from build123d import *

# Parameters (mm, degrees)
BOSS_EXTRUDE1_DEPTH = 20
MOVE_FACE1_BY       = 10
MOVE_FACE2_BY       = 10
SKETCH2_R           = 0.75
CUT_EXTRUDE1_DEPTH  = 88.464278423
SKETCH3_R           = 0.75
CUT_EXTRUDE2_DEPTH  = 108.819293264
SKETCH5_R           = 3.175
CUT_EXTRUDE3_DEPTH  = 88.464278423


with BuildPart() as part:
    # Sketch1 → Boss-Extrude1 (new, symmetric)
    with BuildSketch(Plane.XY):
        Polygon((0, 0), (-40, 0), (-40, 4), (-5, 4), (-5, 55), (50, 55), (50, 50), (0, 50), align=None)
    extrude(amount=BOSS_EXTRUDE1_DEPTH, both=True)

    # Move Face1: a face moved outward by 10.0
    extrude(part.faces().sort_by_distance((22.5, 55, 0))[0], amount=MOVE_FACE1_BY, dir=(0, 1, 0))

    # Move Face2: a face moved inward by 10.0
    extrude(part.faces().sort_by_distance((25, 50, 0))[0], amount=MOVE_FACE2_BY, dir=(0, 1, 0), mode=Mode.SUBTRACT)

    # Sketch2 → Cut-Extrude1 (cut, through all)
    with BuildSketch(Plane.ZY.offset(5)):
        with Locations((-10, 22)):
            Circle(SKETCH2_R)
        with Locations((10, 22)):
            Circle(SKETCH2_R)
        with Locations((10, 47)):
            Circle(SKETCH2_R)
        with Locations((-10, 47)):
            Circle(SKETCH2_R)
    extrude(amount=-CUT_EXTRUDE1_DEPTH, mode=Mode.SUBTRACT)

    # Sketch3 → Cut-Extrude2 (cut, through all)
    with BuildSketch(Plane(origin=(0, 65, -50), x_dir=(1, 0, 0), z_dir=(0, -1, 0))):
        with Locations(Location((10, 39.375, 0), (0, 0, 180))):
            Circle(SKETCH3_R)
        with Locations(Location((35, 39.375, 0), (0, 0, 90))):
            Circle(SKETCH3_R)
        with Locations(Location((35, 60.625, 0), (0, 0, 180))):
            Circle(SKETCH3_R)
        with Locations(Location((10, 60.625, 0), (0, 0, 90))):
            Circle(SKETCH3_R)
    extrude(amount=CUT_EXTRUDE2_DEPTH, mode=Mode.SUBTRACT)

    # Sketch5 → Cut-Extrude3 (cut, through all)
    with BuildSketch(Plane.ZY.offset(5)):
        with Locations(Location((0, 35, 0), (0, 0, 270))):
            Circle(SKETCH5_R)
    extrude(amount=-CUT_EXTRUDE3_DEPTH, mode=Mode.SUBTRACT)


solid = part.part
Could you check a few things on this model? Use its own coordinates, in mm. A direction names the side the tool comes from. Round coordinates to 2 decimals unless told otherwise and drop trailing zeros. Order: outer loops, then holes, each group sorted by start corner. A loop starts at its lowest first (then second) coordinate and runs counter-clockwise, first axis right, second up.
(1) Imagine slicing it at C-C (x = 2). Write out the boundary of the cut face in (y, z), plus the area to 3 significant figures.
Response values:
outline: (60, -20) - (65, -20) - (65, 20) - (60, 20) - close
area: 200 mm2
(2) Imagine slicing it at D-D (y = 13.5). Write out the boundary of the cut face in (x, z).
Response values:
outline: (-5, -20) - (0, -20) - (0, 20) - (-5, 20) - close
(3) Which directions (+Z, -Z, +X, -X, +Y, -Y) give clear straight access to the entire face, cutting with the end or side of a thin tool? Please do faces 1 (the flat face through (25, 60, 0)), 2 (the flat face through (-20, 0, 0)), 3 (the flat face through (-5, 34, -4)).
Response values:
face 1: +Z, -Z, +X, -Y
face 2: +Z, -Z, +X, -X, -Y
face 3: +Z, -Z, -X, +Y
(4) Imagine slicing it at B-B (y = 36). Write out the boundary of the cut face in (x, z), plus the area to 3 significant figures.
Response values:
outline: (-5, -20) - (0, -20) - (0, -3.01) - (-5, -3.01) - close; (-5, 3.01) - (0, 3.01) - (0, 20) - (-5, 20) - close
area: 170 mm2
(5) Imagine slicing it at A-A (z = 14.5). Write out the boundary of the cut face in (x, y).
Response values:
outline: (-40, 0) - (0, 0) - (0, 60) - (50, 60) - (50, 65) - (-5, 65) - (-5, 4) - (-40, 4) - close
(6) I'm going to push flat-ended pins straight in: pin 1 (2 mm diameter, centred on y = 22, z = 10, fed in from +X); pin 2 (7.5 mm diameter, centred on y = 35, z = 0, fed in from -X); pin 3 (2 mm diameter, centred on x = 10, z = -10.625, fed in from -Y). Where does each tip first touch, or does it pass through?
Response values:
pin 1: stops at x = 0
pin 2: stops at x = -5
pin 3: stops at y = 60
(7) If we mould it in two halves opening along Y, with no side actions, what happens to faces 4 (the cylindrical face through (-2.54, 31.97, 0.95)), 5 (the flat face through (-2, 35, -20)), 6 (the flat face through (22, 65, 0))? For each: released by +Y, released by -Y, zero draft, split by the parting line, or undercut.
Response values:
face 4: undercut
face 5: zero draft
face 6: released by +Y
(8) Please list where these lines run through material, in increasing order: line 1 along Z through (x, y) = (-3, 47); line 2 along Y through (x, z) = (-1, -10); line 3 along Y through (x, z) = (-11, -16).
Response values:
line 1: z = -20 to -10.75, -9.25 to 9.25, 10.75 to 20
line 2: y = 0 to 21.25, 22.75 to 46.25, 47.75 to 65
line 3: y = 0 to 4
